from build123d import *

# Parameters (mm, degrees)
F0_W     = 127
F0_H     = 101.6
F1_DEPTH = 6.35
F4_R     = 5.08
F5_DEPTH = 25.4


with BuildPart() as f1:
    # F0 (on Top) → F1 (new body)
    with BuildSketch(Plane.XY):
        Rectangle(F0_W, F0_H)
    extrude(amount=F1_DEPTH)

    # F4
    f4_edges = [f1.edges().sort_by_distance(p)[0] for p in [
        (63.5, 0, 6.35),
        (-63.5, 0, 6.35),
    ]]
    fillet(f4_edges, radius=F4_R)

    # F3 (on offset) → F5 (join)
    with BuildSketch(Plane.XZ.offset(25.4)):
        with BuildLine():
            Line((-50.8, 6.127627), (50.8, 6.127627))
            Line((50.8, 6.127627), (50.8, 56.927627))
            Line((50.8, 56.927627), (12.7, 56.927627))
            ThreePointArc((12.7, 56.927627), (0, 44.227627), (-12.7, 56.927627))
            Line((-12.7, 56.927627), (-50.8, 56.927627))
            Line((-50.8, 56.927627), (-50.8, 6.127627))
        make_face()
    extrude(amount=F5_DEPTH)

    # F6: F1 across plane


with BuildPart() as f1_1:
    add(f1.part)
    add(f1.part.mirror(Plane.XZ))


solid = f1_1.part
Input: part model. Units: mm. Frame: model coordinates. A direction names the side the tool comes from. Give positions to 0.01 mm unless a question says otherwise; leave off trailing zeros. Write each loop counter-clockwise with the first axis right and the second up, starting at its lowest first coordinate (ties: lowest second). Pieces come first, ordered by that corner, then holes.
Q1. Section B-B, the plane x = -27.5. Output: boundary loops of the cut face in (y, z), plus the area to 3 significant figures.
Q2. Section D-D, the plane z = 49. Output: boundary loops of the cut face in (x, y), plus the area to 3 significant figures.
Q3. Set-up query: faces 4 (the face through (-1, 25.4, 32)), 5 (the face through (-1, 1, 0)), 6 (the face through (32, -38, 56.928)), 7 (the face through (50.8, -38, 31)), 8 (the face through (-50.8, 38, 32)). Return all of +Z, -Z, +X, -X, +Y, -Y with unobstructed straight access to the full face (end or side cutting, diameter ignored); none if empty.
Q4. Pull-direction query (X, two-part tool) for faces 1 (the face through (-1, -50.8, 28)), 2 (the face through (-62.051, 0.711, 4.822)), 3 (the face through (0.28, 37.92, 44.23)); classes: pulls with the +X half, pulls with the -X half, needs draft (parallel to the pull), parting line crosses it, or undercut.
Q5. First-contact query: P1, Ø20.5, axis at y = -42, z = 34, coming from the +X side; P2, Ø20.5, axis at y = -41, z = 43, coming from the -X side; P3, Ø2, axis at x = 4, y = -30, coming from the +Z side; P4, Ø6, axis at y = -16, z = 10.5, coming from the +X side. Flat tips, straight axial feed; report the tip coordinate or a pass-through.
Q6. Section A-A, the plane z = 19. Output: boundary loops of the cut face in (x, y), plus the area to 3 significant figures.
Q7. Material intervals for probe 1 along Y at (x, z) = (-38.5, 9); probe 2 along X at (y, z) = (37, 19.5); probe 3 along Z at (x, y) = (28.5, 13), sorted ascending.
Q8. Section C-C, the plane y = -41. Output: boundary loops of the cut face in (x, z).
Filled in:
1. outline: (-50.8, 0) - (50.8, 0) - (50.8, 56.93) - (25.4, 56.93) - (25.4, 6.35) - (-25.4, 6.35) - (-25.4, 56.93) - (-50.8, 56.93) - close
1. area: 3,210 mm2
2. outline: (-50.8, -50.8) - (-9.92, -50.8) - (-9.92, -25.4) - (-50.8, -25.4) - close; (-50.8, 25.4) - (-9.92, 25.4) - (-9.92, 50.8) - (-50.8, 50.8) - close; (9.92, -50.8) - (50.8, -50.8) - (50.8, -25.4) - (9.92, -25.4) - close; (9.92, 25.4) - (50.8, 25.4) - (50.8, 50.8) - (9.92, 50.8) - close
2. area: 4,150 mm2
3. face 4: +Z, +X, -X
3. face 5: -Z, +X, -X, +Y, -Y
3. face 6: +Z, +X, -X, +Y, -Y
3. face 7: +Z, +X, +Y, -Y
3. face 8: +Z, -X, +Y, -Y
4. face 1: needs draft
4. face 2: pulls with the -X half
4. face 3: undercut
5. P1: stops at x = 50.8
5. P2: stops at x = -50.8
5. P3: stops at z = 45.25
5. P4: passes through
6. outline: (-50.8, -50.8) - (50.8, -50.8) - (50.8, -25.4) - (-50.8, -25.4) - close; (-50.8, 25.4) - (50.8, 25.4) - (50.8, 50.8) - (-50.8, 50.8) - close
6. area: 5,160 mm2
7. probe 1: y = -50.8 to -25.4, 25.4 to 50.8
7. probe 2: x = -50.8 to 50.8
7. probe 3: z = 0 to 6.35
8. outline: (-63.5, 0) - (63.5, 0) - (63.5, 1.27) arc R5.08 ccw to (58.42, 6.35) - (50.8, 6.35) - (50.8, 56.93) - (12.7, 56.93) arc R12.7 cw to (-12.7, 56.93) - (-50.8, 56.93) - (-50.8, 6.35) - (-58.42, 6.35) arc R5.08 ccw to (-63.5, 1.27) - close
